The figure shows three views and two pictorial views of one solid part (mm, origin at its lowest corner). Answer the questions. Coordinates: 2 decimals unless noted, no trailing zeros. Order: outer loops, then holes, each group sorted by start corner. A loop starts at its lowest first (then second) coordinate and runs counter-clockwise, first axis right, second up. Notation, with made-up numbers: (19.5, -7.5) -> (52.5, -7.5) arc R34 ccw to (52.5, 23.5) -> close; hole circle Ø6 at (66, 45). An arc over 180 degrees is marked (long way). Return JSON: item names as keys, results as strings.
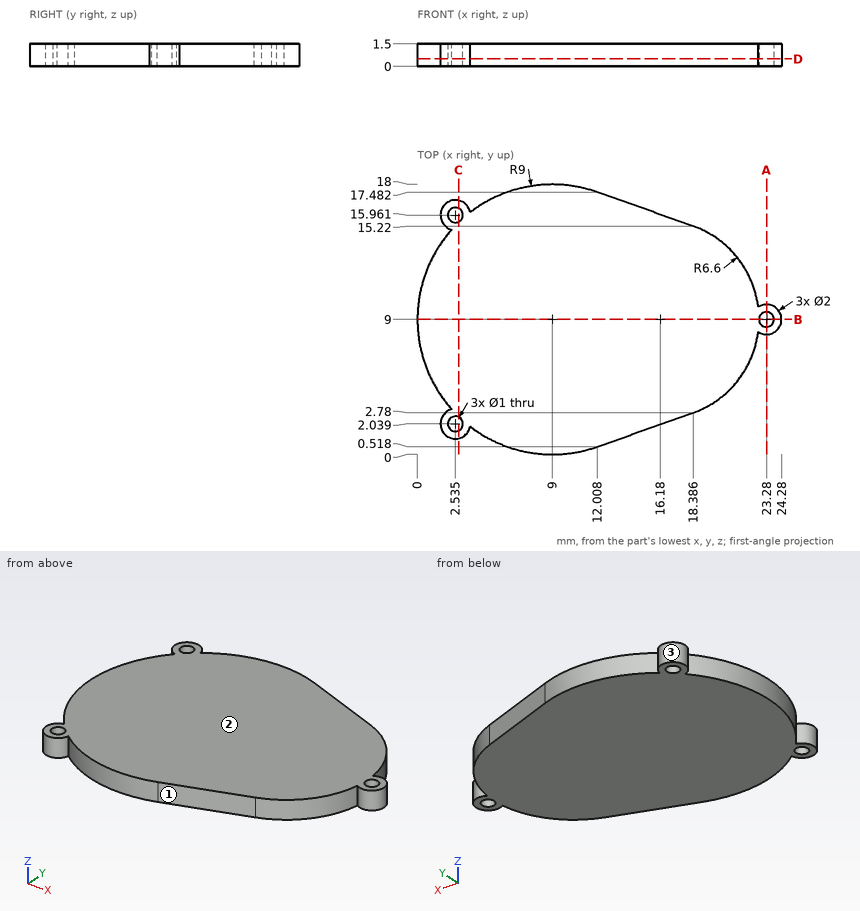
1. Determine the mould class of the marked faces 1, 2 and 3 for opening direction Y: pulls with the +Y half, pulls with the -Y half, needs draft (parallel to the pull), parting line crosses it, or undercut.
Answer block:
{"face 1": "pulls with the -Y half", "face 2": "needs draft", "face 3": "undercut"}
2. The part is cut by section C-C on x = 2.75. Give the vertices of the cut face in (y, z), and give its area (3 significant figures).
Answer block:
{"outline": "(1.06, 0) -> (1.59, 0) -> (1.59, 1.5) -> (1.06, 1.5) -> close; (2.49, 0) -> (15.51, 0) -> (15.51, 1.5) -> (2.49, 1.5) -> close; (16.41, 0) -> (16.94, 0) -> (16.94, 1.5) -> (16.41, 1.5) -> close", "area": "21.1 mm2"}
3. The part is cut by section D-D on z = 0.5. Give the vertices of the cut face in (x, y) (1 decimal), and give its area (3 significant figures).
Answer block:
{"outline": "(2.3, 3) arc R1 ccw (long way) to (3.5, 1.9) arc R9 ccw to (12, 0.5) -> (18.4, 2.8) arc R6.6 ccw to (22.7, 8.2) arc R1 ccw (long way) to (22.7, 9.8) arc R6.6 ccw to (18.4, 15.2) -> (12, 17.5) arc R9 ccw to (3.5, 16.1) arc R1 ccw (long way) to (2.3, 15) arc R9 ccw to start; hole circle Ø1 at (2.5, 2); hole circle Ø1 at (2.5, 16); hole circle Ø1 at (23.3, 9)", "area": "319 mm2"}
4. This flat-tipped pin is pushed along its axis until it touches: pin 1 Ø4 at (x, y) = (16, 5) entering from -Z. Where does it stop, or does it pass through?
Answer block:
{"pin 1": "stops at z = 0"}
5. The part is cut by section B-B on y = 9. Give the vertices of the cut face in (x, z).
Answer block:
{"outline": "(0, 0) -> (22.78, 0) -> (22.78, 1.5) -> (0, 1.5) -> close; (23.78, 0) -> (24.28, 0) -> (24.28, 1.5) -> (23.78, 1.5) -> close"}
6. Consider line 1 (Y direction, x = 2.5, z = 0.5); line 2 (Y direction, x = 8.75, z = 0.45); line 3 (Y direction, x = 1.75, z = 0.15) (1 decimal). Determine where each line is inside the solid, lowest interval first. Write a range as from..to.
Answer block:
{"line 1": "y = 1.04..1.54, 2.54..15.46, 16.46..16.96", "line 2": "y = 0..18", "line 3": "y = 1.4..2.7, 3.7..14.3, 15.3..16.6"}
7. The part is cut by section A-A on x = 23.28. Give the vertices of the cut face in (y, z).
Answer block:
{"outline": "(8, 0) -> (8.5, 0) -> (8.5, 1.5) -> (8, 1.5) -> close; (9.5, 0) -> (10, 0) -> (10, 1.5) -> (9.5, 1.5) -> close"}
